Source: CAD feature listing. Evaluate the final solid. Frame: model axes, mm. Give positions to 0.01 mm unless a question says otherwise; leave off trailing zeros. Write each loop counter-clockwise with the first axis right and the second up, starting at its lowest first coordinate (ties: lowest second). Pieces come first, ordered by that corner, then holes. Notation, with made-up numbers: M 15.25,69.25 L 71.25,69.25 A16 cw 71.25,74.25 Z; hole C 37.5,86 d1. An arc over 180 degrees is marked long. Return JSON: item names as keys, results as strings.
```python
from build123d import *

# Parameters (mm, degrees)
F0_R     = 2.5
F1_DEPTH = 2.5


with BuildPart() as f1:
    # F0 (on Top) → F1 (new body)
    with BuildSketch(Plane.XY):
        with BuildLine():
            Line((0, -20), (0, 20))
            Line((0, 20), (-5, 15))
            ThreePointArc((-5, 15), (-12.803301, -7.196699), (-35, -15))
            Line((-35, -15), (-40, -20))
            Line((-40, -20), (0, -20))
        make_face()
        with Locations((-7.5, -12.5)):
            Circle(F0_R, mode=Mode.SUBTRACT)
    extrude(amount=F1_DEPTH)

    # F2: F1 across face


with BuildPart() as f1_1:
    add(f1.part)
    add(f1.part.mirror(Plane(origin=(0, 0, 1.25), x_dir=(0, 1, 0), z_dir=(1, 0, 0))))


solid = f1_1.part
```
1) Cut plane C-C, the plane y = -12.5. Return the cut outline in (x, z).
Numbers:
{"outline": "M -20.3,0 L -10,0 L -10,2.5 L -20.3,2.5 Z; M -5,0 L 5,0 L 5,2.5 L -5,2.5 Z; M 10,0 L 20.3,0 L 20.3,2.5 L 10,2.5 Z"}
2) Cut plane D-D, the plane y = 8. Return the cut outline in (x, z), then the cut area to 3 significant figures.
Numbers:
{"outline": "M -5.14,0 L 5.14,0 L 5.14,2.5 L -5.14,2.5 Z", "area": "25.7 mm²"}
3) Contact query for flat-ended pins moving along their axis: pin 1 Ø3 at (x, y) = (-7.5, -12.5) entering from +Z; pin 2 Ø1.5 at (y, z) = (6, 1.5) entering from +X; pin 3 Ø1 at (x, z) = (10, 1.5) entering from +Y. Output: stop coordinate, or through.
Numbers:
{"pin 1": "passes through", "pin 2": "stops at x = 5.7", "pin 3": "stops at y = -3.19"}
4) Cut plane A-A, the plane z = 1. Return the cut outline in (x, y), then the cut area to 3 significant figures.
Numbers:
{"outline": "M -40,-20 L 40,-20 L 35,-15 A27.2 cw 5,15 L 0,20 L -5,15 A27.2 cw -35,-15 Z; hole C -7.5,-12.5 d5; hole C 7.5,-12.5 d5", "area": "959 mm²"}
5) Line query: line 1 (Y direction, x = -7.5, z = 1.95); line 2 (Y direction, x = -32, z = 0.75); line 3 (X direction, y = 7, z = 0.4). Output: solid intervals per line, ascending. Write a range as [from, to].
Numbers:
{"line 1": "y = [-20, -15], [-10, 0.3]", "line 2": "y = [-20, -15.16]", "line 3": "x = [-5.31, 5.31]"}
6) Cut plane B-B, the plane x = -7.5. Return the cut outline in (y, z), then the cut area to 3 significant figures.
Numbers:
{"outline": "M -20,0 L -15,0 L -15,2.5 L -20,2.5 Z; M -10,0 L 0.3,0 L 0.3,2.5 L -10,2.5 Z", "area": "38.2 mm²"}
